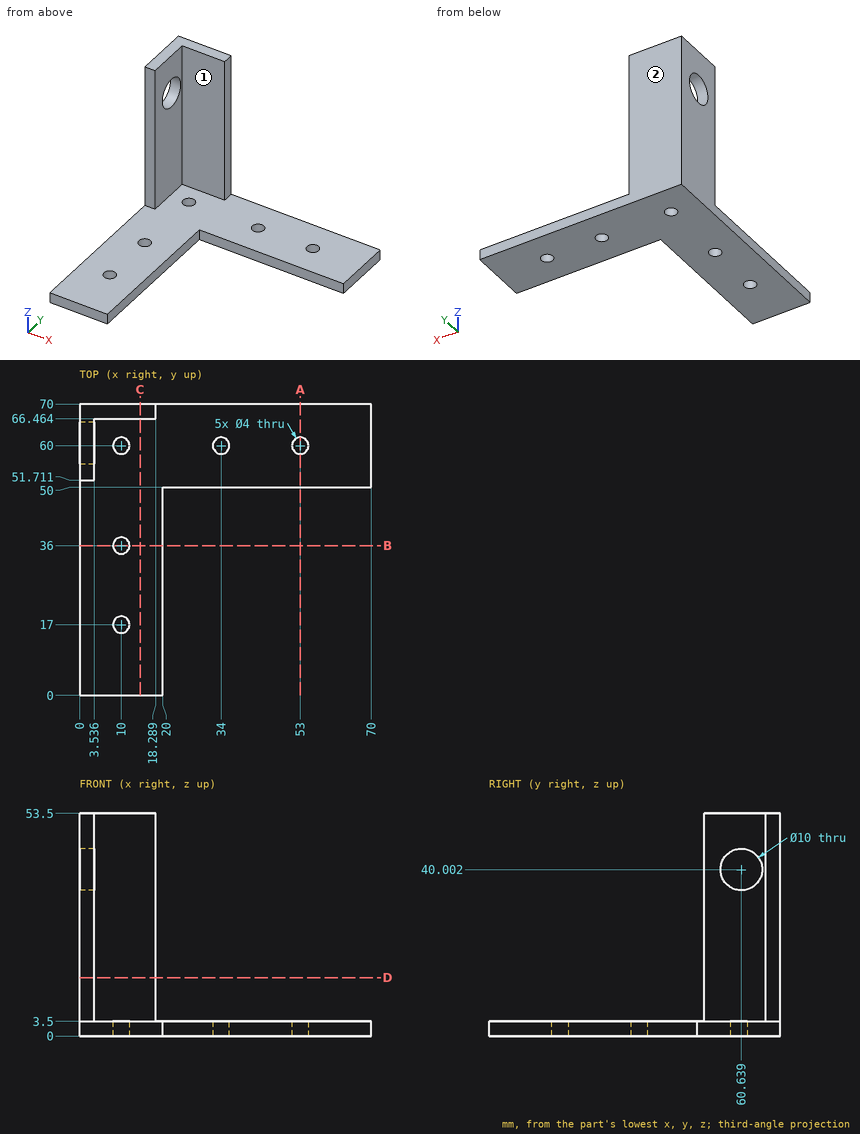
Job drawing, mm, ordinate dimensions from the low corner. One solid piece. A direction names the side the tool comes from. Round coordinates to 2 decimals unless told otherwise and drop trailing zeros. Write each loop counter-clockwise with the first axis right and the second up, starting at its lowest first coordinate (ties: lowest second). Pieces come first, ordered by that corner, then holes. Notation, with made-up numbers: M 55,-24.5 L 81,-24.5 A33 cw 81,13.5 Z; hole C -28.5,29 d11. An arc over 180 degrees is marked long. Return JSON: item names as keys, results as strings. Group by question number.
(1) Drill centre lines: probe 1 along Y at (x, z) = (10, 1); probe 2 along Y at (x, z) = (34, 2); probe 3 along X at (y, z) = (53, 32) (1 decimal). Where is each one in solid material? Low to high.
(2) Saw through at A-A on x = 53. Write the cut outline in (y, z).
(3) Saw through at D-D on z = 14. Write the cut outline in (x, y) (1 decimal), then the cut area to 3 significant figures.
(4) Which spindle directions (+Z, -Z, +X, -X, +Y, -Y) get a long thin tool onto all of the face, cutting with end or side? Do the marked faces 1 and 2. Say none if no direction does.
(5) Pin check, flat tips, straight feed: pin 1 Ø10 at (y, z) = (48, 29) entering from +X; pin 2 Ø1.8 at (x, z) = (1.5, 36) entering from -Y; pin 3 Ø1 at (y, z) = (23, 2) entering from +X. Stop position of each tip, or through.
(6) Saw through at B-B on y = 36. Write the cut outline in (x, z), then the cut area to 3 significant figures.
(7) Saw through at C-C on x = 14.5. Write the cut outline in (y, z) (1 decimal), then the cut area to 3 significant figures.
Returned:
{
 "1": {"probe 1": "0 to 15, 19 to 34, 38 to 58, 62 to 70", "probe 2": "50 to 58, 62 to 70", "probe 3": "0 to 3.5"},
 "2": {"outline": "M 50,0 L 58,0 L 58,3.5 L 50,3.5 Z; M 62,0 L 70,0 L 70,3.5 L 62,3.5 Z"},
 "3": {"outline": "M 0,51.7 L 3.5,51.7 L 3.5,66.5 L 18.3,66.5 L 18.3,70 L 0,70 Z", "area": "117 mm²"},
 "4": {"face 1": "+Z, +X, -Y", "face 2": "+Z, -Z, +X, -X, +Y"},
 "5": {"pin 1": "x = 3.54", "pin 2": "y = 51.71", "pin 3": "x = 20"},
 "6": {"outline": "M 0,0 L 8,0 L 8,3.5 L 0,3.5 Z; M 12,0 L 20,0 L 20,3.5 L 12,3.5 Z", "area": "56.0 mm²"},
 "7": {"outline": "M 0,0 L 70,0 L 70,53.5 L 66.5,53.5 L 66.5,3.5 L 0,3.5 Z", "area": "422 mm²"}
}
